Can you work these out from the model? Positions are in its coordinate system, mm. A direction names the side the tool comes from. Round coordinates to 2 decimals unless told otherwise and drop trailing zeros. Loops run counter-clockwise (first coordinate to the right, second up) from the corner with the lowest first, then second, coordinate; pieces in that order, holes last.
(1) I want a section at D-D on y = 2.5. Write out the boundary of the cut face in (x, z).
(2) Will these pins go through, and if not, where does the flat tip stop? pin 1 Ø3.5 at (y, z) = (16.5, 14.91) entering from -X; pin 2 Ø8 at (x, y) = (-5.5, 17) entering from +Z.
(3) Thinking about a two-plate mould opening in Y: for faces 3 (the face through (-24, 2, 0)), 4 (the face through (-38.666, -13.71, -0.394)), 5 (the face through (0.29, 16.15, 31.74)), 6 (the face through (0.29, -14.68, 15.99)), which applies, released by +Y, released by -Y, zero draft, split by the parting line, or undercut?
(4) I want a section at B-B on x = -33.4. Write out the boundary of the cut face in (y, z).
(5) I want a section at A-A on y = 16.5. Write out the boundary of the cut face in (x, z).
(6) I want a section at C-C on y = -13.5. Write out the boundary of the cut face in (x, z), plus the area to 3 significant figures.
(7) Which directions (+Z, -Z, +X, -X, +Y, -Y) give clear straight access to the entire face, cutting with the end or side of a thin tool? Please do faces 1 (the face through (-14.15, 17.85, -0.39)), 2 (the face through (-0.1, 1, 25)).
(8) If I drill on line 1 along Z through (x, y) = (0, 16); line 2 along Z through (x, y) = (0.55, 16.5); line 3 along X through (y, z) = (17.5, 44), over which ranges is the centre line in solid material (lowest first)?
from build123d import *

# Parameters (mm, degrees)
SKETCH3_R                  = 1.6
BASE_FLANGE1_DEPTH         = 0.8
SKETCHED_START             = 0.510326571
SKETCHED_BEND1_OUTLINE_W   = 60
SKETCHED_BEND1_OUTLINE_H   = 0.8
SKETCHED_BEND1_DEPTH       = 47.889673429
SKETCHED_START_2           = -1.099557429
SKETCHED_BEND1_2_OUTLINE_R = 1.6
SKETCHED_BEND1_2_DEPTH     = 1.8
SKETCHED_START_3           = -28.5
SKETCHED_BEND1_3_DEPTH     = 60


with BuildPart() as part:
    # Base-Flange1: sheet metal written as solids
    # Sketch3 → Base-Flange1 (new body)
    with BuildSketch(Plane.XY):
        Polygon((29.2, -28.5), (-29.2, -28.5), (-48.4, 1.5), (-48.4, 31.5), (48.4, 31.5), (48.4, 1.5), align=None)
        with Locations((-33.4, 16.5)):
            Circle(SKETCH3_R, mode=Mode.SUBTRACT)
        with Locations((-15.009973435, 16.5)):
            Circle(SKETCH3_R, mode=Mode.SUBTRACT)
        with Locations((-15.009973435, -13.5)):
            Circle(SKETCH3_R, mode=Mode.SUBTRACT)
        with Locations(Location((15.009973435, -13.5, 0), (0, 0, 180))):
            Circle(SKETCH3_R, mode=Mode.SUBTRACT)
        with Locations(Location((15.009973435, 16.5, 0), (0, 0, 180))):
            Circle(SKETCH3_R, mode=Mode.SUBTRACT)
        with Locations(Location((33.4, 16.5, 0), (0, 0, 180))):
            Circle(SKETCH3_R, mode=Mode.SUBTRACT)
    extrude(amount=-BASE_FLANGE1_DEPTH)

    # Sketched Bend1: read off the stored shape, not the designer's step
    # Sketched Bend1 outline → Sketched Bend1 (cut)
    with BuildSketch(Plane.YZ.offset(SKETCHED_START)):
        with Locations((1.5, -0.4)):
            Rectangle(SKETCHED_BEND1_OUTLINE_W, SKETCHED_BEND1_OUTLINE_H)
    extrude(amount=SKETCHED_BEND1_DEPTH, mode=Mode.SUBTRACT)

    # Sketched Bend1 2 outline → Sketched Bend1 2 (add)
    with BuildSketch(Plane.YZ.offset(SKETCHED_START_2)):
        Polygon((31.5, 0), (31.5, 48.300442571), (1.5, 48.300442571), (-28.5, 29.100442571), (-28.5, 0), align=None)
        with Locations((-13.5, 14.910416006)):
            Circle(SKETCHED_BEND1_2_OUTLINE_R, mode=Mode.SUBTRACT)
        with Locations((16.5, 14.910416006)):
            Circle(SKETCHED_BEND1_2_OUTLINE_R, mode=Mode.SUBTRACT)
        with Locations((16.5, 33.300442571)):
            Circle(SKETCHED_BEND1_2_OUTLINE_R, mode=Mode.SUBTRACT)
    extrude(amount=SKETCHED_BEND1_2_DEPTH)

    # Sketched Bend1 3 outline → Sketched Bend1 3 (cut)
    with BuildSketch(Plane(origin=(0, 0, 0), x_dir=(1, 0, 0), z_dir=(0, 1, 0)).offset(SKETCHED_START_3)):
        with BuildLine():
            Line((-1.099557429, -48.300442571), (-0.099557429, -48.300442571))
            Line((-0.099557429, -48.300442571), (-0.099557429, -1))
            ThreePointArc((-0.099557429, -1), (-0.392450648, -0.292893219), (-1.099557429, 0))
            Line((-1.099557429, 0), (-1.099557429, -48.300442571))
        make_face()
        with BuildLine():
            ThreePointArc((-1.099557429, 0.8), (0.173234777, 0.272792206), (0.700442571, -1))
            Line((0.700442571, -1), (0.700442571, 0))
            Line((0.700442571, 0), (0.510326571, 0))
            Line((0.510326571, 0), (0.510326571, 0.8))
            Line((0.510326571, 0.8), (-1.099557429, 0.8))
        make_face()
    extrude(amount=SKETCHED_BEND1_3_DEPTH, mode=Mode.SUBTRACT)


solid = part.part
Filled sheet:
1. outline: (-48.4, -0.8) - (-1.1, -0.8) arc R1.8 ccw to (0.7, 1) - (0.7, 48.3) - (-0.1, 48.3) - (-0.1, 1) arc R1 cw to (-1.1, 0) - (-48.4, 0) - close
2. pin 1: stops at x = -0.1
2. pin 2: stops at z = 0
3. face 3: zero draft
3. face 4: released by -Y
3. face 5: undercut
3. face 6: undercut
4. outline: (-21.94, -0.8) - (14.9, -0.8) - (14.9, 0) - (-21.94, 0) - close; (18.1, -0.8) - (31.5, -0.8) - (31.5, 0) - (18.1, 0) - close
5. outline: (-48.4, -0.8) - (-35, -0.8) - (-35, 0) - (-48.4, 0) - close; (-31.8, -0.8) - (-16.61, -0.8) - (-16.61, 0) - (-31.8, 0) - close; (-13.41, -0.8) - (-1.1, -0.8) arc R1.8 ccw to (0.7, 1) - (0.7, 13.31) - (-0.1, 13.31) - (-0.1, 1) arc R1 cw to (-1.1, 0) - (-13.41, 0) - close; (-0.1, 16.51) - (0.7, 16.51) - (0.7, 31.7) - (-0.1, 31.7) - close; (-0.1, 34.9) - (0.7, 34.9) - (0.7, 48.3) - (-0.1, 48.3) - close
6. outline: (-38.8, -0.8) - (-16.61, -0.8) - (-16.61, 0) - (-38.8, 0) - close; (-13.41, -0.8) - (-1.1, -0.8) arc R1.8 ccw to (0.7, 1) - (0.7, 13.31) - (-0.1, 13.31) - (-0.1, 1) arc R1 cw to (-1.1, 0) - (-13.41, 0) - close; (-0.1, 16.51) - (0.7, 16.51) - (0.7, 38.7) - (-0.1, 38.7) - close
6. area: 57.0 mm2
7. face 1: +Z, -Z
7. face 2: +Z, -X, +Y, -Y
8. line 1: z = -0.43 to 13.39, 16.43 to 31.78, 34.82 to 48.3
8. line 2: z = 0.28 to 13.31, 16.51 to 31.7, 34.9 to 48.3
8. line 3: x = -0.1 to 0.7
